Model file for the job. Use its own axes, mm. Face numbers are marked on the shaded views. A direction names the side the tool comes from. Give positions to 0.01 mm unless a question says otherwise; leave off trailing zeros. Loops run counter-clockwise (first coordinate to the right, second up) from the corner with the lowest first, then second, coordinate; pieces in that order, holes last. Notation, with made-up numbers: M 11,-24.75 L 59,-24.75 A10 ccw 59,-9.75 Z; hole C 10.25,3 d8. An arc over 180 degrees is marked long. Answer in a Markdown table with one row per item.
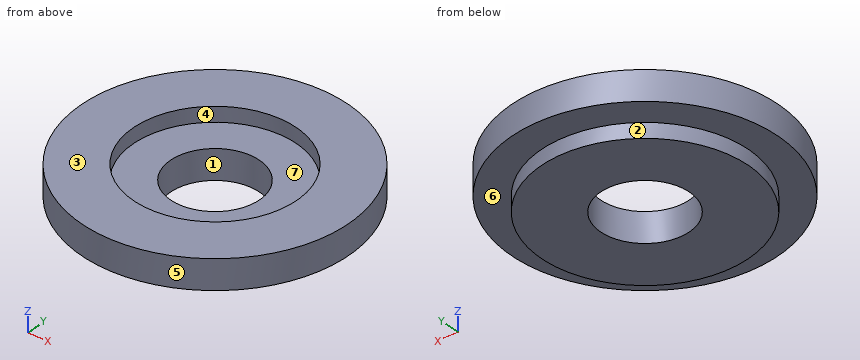
Autodesk Inventor part; units mm, degrees
ref_plane "YZ Plane" through (0, 0, 0) normal (1, 0, 0) x (0, 1, 0)
ref_plane "XZ Plane" through (0, 0, 0) normal (0, 1, 0) x (-1, 0, 0)
ref_plane "XY Plane" through (0, 0, 0) normal (0, 0, 1) x (1, 0, 0)
sketch "Skizze1" plane through (0, 0, 0) normal (0, 1, 0) x (-1, 0, 0)
  line L0 (0, 0) -> (4.5, 0)
  line L1 (4.5, 0) -> (4.5, -1)
  line L2 (4.5, -1) -> (3.5, -1)
  line L3 (3.5, -1) -> (3.5, -1.5)
  line L4 (3.5, -1.5) -> (0, -1.5)
  line L5 (0, -1.5) -> (0, 0)
  point P0 (4.5, -0.5)
  dimension "d0" = 1.5
  dimension "d1" = 0.5
  dimension "d2" = 9
  dimension "d3" = 7
revolve "Umdrehung1" add sketch "Skizze1" angle 360 about axis through (0, 0, -1.5) along (0, 0, 1)
sketch "Skizze3" plane through (0, 0, 0) normal (1, 0, 0) x (0, 1, 0)
  line L0 (0, 0) -> (2.75, 0)
  line L1 (4.5, 0) -> (-4.5, 0)
  line L2 (2.75, 0) -> (2.75, -0.5)
  line L3 (2.75, -0.5) -> (1.5, -0.5)
  line L4 (1.5, -0.5) -> (1.5, -1.5)
  line L5 (1.5, -1.5) -> (0, -1.5)
  line L6 (0, -1.5) -> (0, 0)
  line L7 (3.5, -1.5) -> (-3.5, -1.5)
  dimension "d5" = 3
  dimension "d6" = 5.5
  dimension "d7" = 0.5
revolve "Umdrehung2" cut sketch "Skizze3" angle 360 about axis through (0, 0, -1.5) along (0, 0, 1)
properties part number "Miederhalter_ventilfeder"
Q1. Mould opens along X. For the marked faces 1, 2, 3 and 4 say: released by +X, released by -X, zero draft, split by the parting line, or undercut.
Reported:
| item | result |
|---|---|
| face 1 | undercut |
| face 2 | split by the parting line |
| face 3 | zero draft |
| face 4 | undercut |
Q2. Saw through at D-D (y = -2.5). Give the cut face in (x, z).
Reported:
| item | result |
|---|---|
| outline | M -3.74,-1 L -2.45,-1 L -2.45,-1.5 L 2.45,-1.5 L 2.45,-1 L 3.74,-1 L 3.74,0 L 1.15,0 L 1.15,-0.5 L -1.15,-0.5 L -1.15,0 L -3.74,0 Z |
Q3. Probe probe 1 along X at (y, z) = (0, -1.05); probe 2 along X at (y, z) = (0, -0.95); probe 3 along Y at (x, z) = (0, -0.3). List the from-to ranges inside material, lowest first.
Reported:
| item | result |
|---|---|
| probe 1 | -3.5 to -1.5, 1.5 to 3.5 |
| probe 2 | -4.5 to -1.5, 1.5 to 4.5 |
| probe 3 | -4.5 to -2.75, 2.75 to 4.5 |
Q4. 3-axis set-ups, long thin cutter, end or side, ignore diameter. For the marked faces 5, 6 and 7: which of +Z, -Z, +X, -X, +Y, -Y reach the whole face in a straight line?
Reported:
| item | result |
|---|---|
| face 5 | +Z, -Z |
| face 6 | -Z |
| face 7 | +Z |
Q5. Saw through at B-B (x = 0.5). Give the cut face in (y, z), and give its area (3 significant figures).
Reported:
| item | result |
|---|---|
| outline | M -4.47,-1 L -3.46,-1 L -3.46,-1.5 L -1.41,-1.5 L -1.41,-0.5 L -2.7,-0.5 L -2.7,0 L -4.47,0 Z; M 1.41,-1.5 L 3.46,-1.5 L 3.46,-1 L 4.47,-1 L 4.47,0 L 2.7,0 L 2.7,-0.5 L 1.41,-0.5 Z |
| area | 6.88 mm² |
Q6. Drop a flat-ended pin along its axis: pin 1 (1.5 mm diameter, centred on x = 1.5, y = -1, fed in from +Z). Give the stop position or say it passes through.
Reported:
| item | result |
|---|---|
| pin 1 | z = -0.5 |
Q7. Saw through at A-A (y = 0). Give the cut face in (x, z).
Reported:
| item | result |
|---|---|
| outline | M -4.5,-1 L -3.5,-1 L -3.5,-1.5 L -1.5,-1.5 L -1.5,-0.5 L -2.75,-0.5 L -2.75,0 L -4.5,0 Z; M 1.5,-1.5 L 3.5,-1.5 L 3.5,-1 L 4.5,-1 L 4.5,0 L 2.75,0 L 2.75,-0.5 L 1.5,-0.5 Z |
Q8. Saw through at C-C (z = -0.65). Give the cut face in (x, y), and give its area (3 significant figures).
Reported:
| item | result |
|---|---|
| outline | C 0,0 d9; hole C 0,0 d3 |
| area | 56.5 mm² |
